Build history of the part. All positions in model axes, mm. Round coordinates to 2 decimals unless told otherwise and drop trailing zeros. Order: outer loops, then holes, each group sorted by start corner. A loop starts at its lowest first (then second) coordinate and runs counter-clockwise, first axis right, second up. Notation, with made-up numbers: (35, -39) -> (86, -39) arc R11 cw to (86, -19) -> close; hole circle Ø8 at (81.25, 53.5). An arc over 180 degrees is marked (long way). Use a Markdown table: item, result. Add a question column.
Item 1: Slice it at C-C, the plane z = -12. Give the cut face in (x, y), plus the area to 3 significant figures.
Item 2: Pin check, flat tips, straight feed: pin 1 (3 mm diameter, centred on x = -23, y = 1, fed in from -Z); pin 2 (1.9 mm diameter, centred on y = 3, z = -19, fed in from -X); pin 3 (2 mm diameter, centred on x = 18, y = 4, fed in from -Z). Stop position of each tip, or through.
Item 3: Slice it at B-B, the plane z = 0. Give the cut face in (x, y) (3 decimals).
Item 4: Slice it at D-D, the plane x = 16. Give the cut face in (y, z), plus the area to 3 significant figures.
Item 5: Slice it at A-A, the plane x = 0. Give the cut face in (y, z) (3 decimals), plus the area to 3 significant figures.
Item 6: Two-plate mould, pull along Z, no slides. Class faces 1 (the face through (12.164, 3.131, -9.919)), 2 (the face through (-6.883, 3.131, 30.995)): released by +Z, released by -Z, zero draft, split by the parting line, or undercut.
Item 7: Probe L1, parallel to X at y = 5, z = 0 (3 decimals); L2, parallel to Z at x = 2, y = 1.75. List the from-to ranges inside material, lowest first.
from build123d import *

# Parameters (mm, degrees)
SKETCH1_R           = 31.75
SKETCH1_R_2         = 3.175
BOSS_EXTRUDE1_DEPTH = 6.35


with BuildPart() as part:
    # Sketch1 → Boss-Extrude1 (new body)
    with BuildSketch(Plane(origin=(0, 0, 0), x_dir=(1, 0, 0), z_dir=(0, 1, 0))):
        Circle(SKETCH1_R)
        with BuildLine():
            Line((-1.5875, -6.148361062), (-1.5875, -25.350342083))
            ThreePointArc((-1.5875, -25.350342083), (-9.720159182, -23.466540126), (-16.802866778, -19.047930808))
            Line((-16.802866778, -19.047930808), (-3.225015785, -5.470079815))
            ThreePointArc((-3.225015785, -5.470079815), (-2.430039796, -5.866635031), (-1.5875, -6.148361062))
        make_face(mode=Mode.SUBTRACT)
        with BuildLine():
            Line((-5.470079815, -3.225015785), (-19.047930808, -16.802866778))
            ThreePointArc((-19.047930808, -16.802866778), (-23.466540126, -9.720159182), (-25.350342083, -1.5875))
            Line((-25.350342083, -1.5875), (-6.148361062, -1.5875))
            ThreePointArc((-6.148361062, -1.5875), (-5.866635031, -2.430039796), (-5.470079815, -3.225015785))
        make_face(mode=Mode.SUBTRACT)
        with BuildLine():
            Line((3.225015785, -5.470079815), (16.802866778, -19.047930808))
            ThreePointArc((16.802866778, -19.047930808), (9.720159182, -23.466540126), (1.5875, -25.350342083))
            Line((1.5875, -25.350342083), (1.5875, -6.148361062))
            ThreePointArc((1.5875, -6.148361062), (2.430039796, -5.866635031), (3.225015785, -5.470079815))
        make_face(mode=Mode.SUBTRACT)
        with BuildLine():
            Line((6.148361062, -1.5875), (25.350342083, -1.5875))
            ThreePointArc((25.350342083, -1.5875), (23.466540126, -9.720159182), (19.047930808, -16.802866778))
            Line((19.047930808, -16.802866778), (5.470079815, -3.225015785))
            ThreePointArc((5.470079815, -3.225015785), (5.866635031, -2.430039796), (6.148361062, -1.5875))
        make_face(mode=Mode.SUBTRACT)
        with BuildLine():
            Line((-6.148361062, 1.5875), (-25.350342083, 1.5875))
            ThreePointArc((-25.350342083, 1.5875), (-23.466540126, 9.720159182), (-19.047930808, 16.802866778))
            Line((-19.047930808, 16.802866778), (-5.470079815, 3.225015785))
            ThreePointArc((-5.470079815, 3.225015785), (-5.866635031, 2.430039796), (-6.148361062, 1.5875))
        make_face(mode=Mode.SUBTRACT)
        with BuildLine():
            ThreePointArc((-16.802866778, 19.047930808), (-9.720159182, 23.466540126), (-1.5875, 25.350342083))
            Line((-1.5875, 25.350342083), (-1.5875, 6.148361062))
            ThreePointArc((-1.5875, 6.148361062), (-2.430039796, 5.866635031), (-3.225015785, 5.470079815))
            Line((-3.225015785, 5.470079815), (-16.802866778, 19.047930808))
        make_face(mode=Mode.SUBTRACT)
        Circle(SKETCH1_R_2, mode=Mode.SUBTRACT)
        with BuildLine():
            Line((5.470079815, 3.225015785), (19.047930808, 16.802866778))
            ThreePointArc((19.047930808, 16.802866778), (23.466540126, 9.720159182), (25.350342083, 1.5875))
            Line((25.350342083, 1.5875), (6.148361062, 1.5875))
            ThreePointArc((6.148361062, 1.5875), (5.866635031, 2.430039796), (5.470079815, 3.225015785))
        make_face(mode=Mode.SUBTRACT)
        with BuildLine():
            Line((3.225015785, 5.470079815), (3.175, 5.42006403))
            Line((3.175, 5.42006403), (3.175, 5.499261314))
            ThreePointArc((3.175, 5.499261314), (2.403265317, 5.877653938), (1.5875, 6.148361062))
            Line((1.5875, 6.148361062), (1.5875, 25.350342083))
            ThreePointArc((1.5875, 25.350342083), (9.720159182, 23.466540126), (16.802866778, 19.047930808))
            Line((16.802866778, 19.047930808), (3.225015785, 5.470079815))
        make_face(mode=Mode.SUBTRACT)
    extrude(amount=BOSS_EXTRUDE1_DEPTH)


solid = part.part
Check sheet entries:
| question | item | result |
|---|---|---|
| 1 | outline | (-29.39, 0) -> (-22.39, 0) -> (-22.39, 6.35) -> (-29.39, 6.35) -> close; (-14.25, 0) -> (-9.75, 0) -> (-9.75, 6.35) -> (-14.25, 6.35) -> close; (-1.59, 0) -> (1.59, 0) -> (1.59, 6.35) -> (-1.59, 6.35) -> close; (9.75, 0) -> (14.25, 0) -> (14.25, 6.35) -> (9.75, 6.35) -> close; (22.39, 0) -> (29.39, 0) -> (29.39, 6.35) -> (22.39, 6.35) -> close |
| 1 | area | 166 mm2 |
| 2 | pin 1 | z = -23.36 |
| 2 | pin 2 | x = -26.12 |
| 2 | pin 3 | z = -26.82 |
| 3 | outline | (-31.75, 0) -> (-3.175, 0) -> (-3.175, 6.35) -> (-31.75, 6.35) -> close; (3.175, 0) -> (31.75, 0) -> (31.75, 6.35) -> (3.175, 6.35) -> close |
| 4 | outline | (0, -27.42) -> (6.35, -27.42) -> (6.35, -19.73) -> (0, -19.73) -> close; (0, -18.25) -> (6.35, -18.25) -> (6.35, -13.75) -> (0, -13.75) -> close; (0, -1.59) -> (6.35, -1.59) -> (6.35, 1.59) -> (0, 1.59) -> close; (0, 13.75) -> (6.35, 13.75) -> (6.35, 18.25) -> (0, 18.25) -> close; (0, 19.73) -> (6.35, 19.73) -> (6.35, 27.42) -> (0, 27.42) -> close |
| 4 | area | 175 mm2 |
| 5 | outline | (0, -31.75) -> (6.35, -31.75) -> (6.35, -3.175) -> (0, -3.175) -> close; (0, 3.175) -> (6.35, 3.175) -> (6.35, 31.75) -> (0, 31.75) -> close |
| 5 | area | 363 mm2 |
| 6 | face 1 | undercut |
| 6 | face 2 | split by the parting line |
| 7 | L1 | -31.75 to -3.175, 3.175 to 31.75 |
| 7 | L2 | -31.69 to -25.32, -6.03 to -2.47, 2.47 to 6.03, 25.32 to 31.69 |
